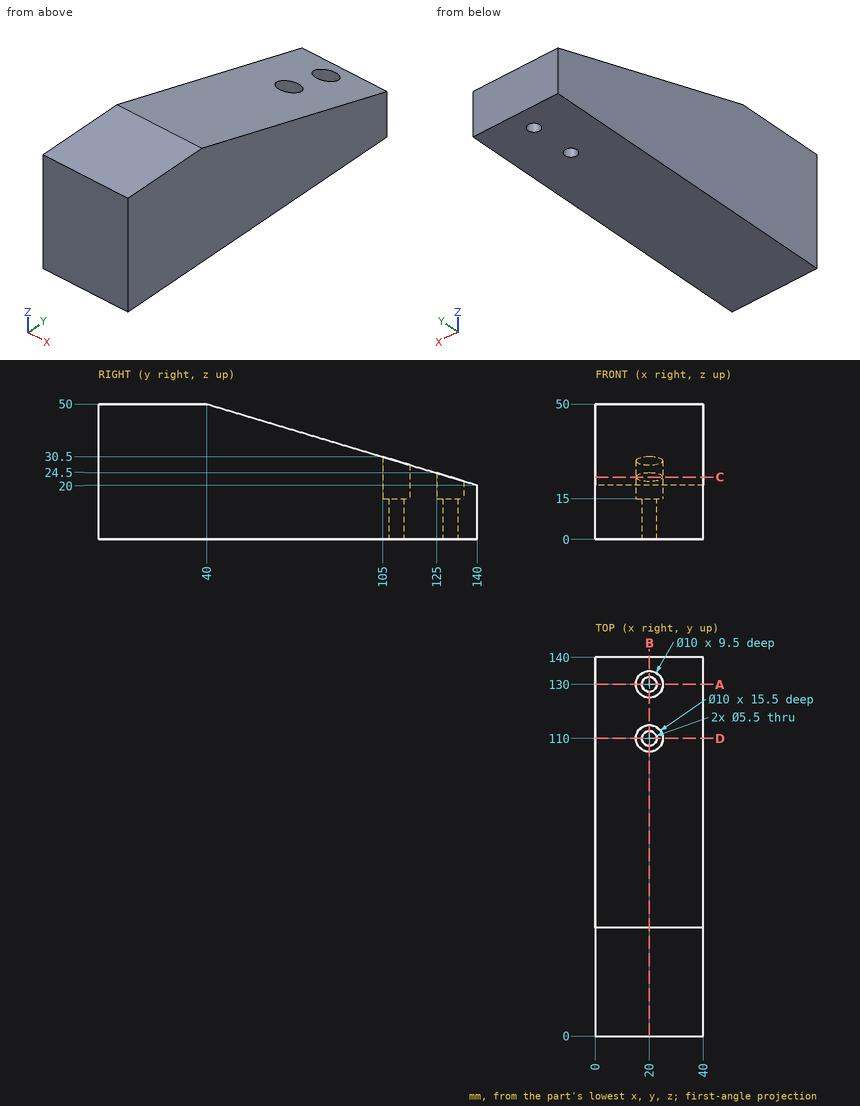
Job drawing, mm, ordinate dimensions from the low corner. One solid piece. Round coordinates to 2 decimals unless told otherwise and drop trailing zeros. Loops run counter-clockwise (first coordinate to the right, second up) from the corner with the lowest first, then second, coordinate; pieces in that order, holes last.
Item 1: Drill centre lines: line 1 (Y direction, x = 20, z = 4.75); line 2 (X direction, y = 130, z = 3.5); line 3 (X direction, y = 110, z = 21). Where is each one in solid material? Low to high.
Item 2: Cut at D-D, the plane y = 110. Give the cut face in (x, z).
Item 3: Drop flat-ended pins along their axis: P1, Ø3, axis at x = 19.5, y = 111, coming from the +Z side; P2, Ø11, axis at x = 18.5, y = 132, coming from the +Z side; P3, Ø8, axis at x = 20, y = 110, coming from the +Z side; P4, Ø12, axis at x = 14.5, y = 72.5, coming from the +Z side. Give the stop position or say it passes through.
Item 4: Cut at A-A, the plane y = 130. Give the cut face in (x, z).
Item 5: Cut at C-C, the plane z = 23. Give the cut face in (x, y).
Item 6: Cut at B-B, the plane x = 20. Give the cut face in (y, z).
A:
1. line 1: y = 0 to 107.25, 112.75 to 127.25, 132.75 to 140
1. line 2: x = 0 to 17.25, 22.75 to 40
1. line 3: x = 0 to 15, 25 to 40
2. outline: (0, 0) - (17.25, 0) - (17.25, 15) - (15, 15) - (15, 29) - (0, 29) - close; (22.75, 0) - (40, 0) - (40, 29) - (25, 29) - (25, 15) - (22.75, 15) - close
3. P1: passes through
3. P2: stops at z = 23.85
3. P3: stops at z = 15
3. P4: stops at z = 42.05
4. outline: (0, 0) - (17.25, 0) - (17.25, 15) - (15, 15) - (15, 23) - (0, 23) - close; (22.75, 0) - (40, 0) - (40, 23) - (25, 23) - (25, 15) - (22.75, 15) - close
5. outline: (0, 0) - (40, 0) - (40, 130) - (25, 130) arc R5 cw to (15, 130) - (0, 130) - close; hole circle Ø10 at (20, 110)
6. outline: (0, 0) - (107.25, 0) - (107.25, 15) - (105, 15) - (105, 30.5) - (40, 50) - (0, 50) - close; (112.75, 0) - (127.25, 0) - (127.25, 15) - (125, 15) - (125, 24.5) - (115, 27.5) - (115, 15) - (112.75, 15) - close; (132.75, 0) - (140, 0) - (140, 20) - (135, 21.5) - (135, 15) - (132.75, 15) - close
